Can you work these out from the model? Positions are in its coordinate system, mm. A direction names the side the tool comes from. Round coordinates to 2 decimals unless told otherwise and drop trailing zeros. One line per question, with ' | ' between items.
```python
from build123d import *

# Parameters (mm, degrees)
SKETCH1_R           = 2.5
BOSS_EXTRUDE1_DEPTH = 200


with BuildPart() as part:
    # Sketch1 → Boss-Extrude1 (new body)
    with BuildSketch(Plane(origin=(0, 0, -25), x_dir=(-1, 0, 0), z_dir=(0, 0, -1))):
        with BuildLine():
            Line((12.5, 4.32), (12.5, 10.537068835))
            ThreePointArc((12.5, 10.537068835), (11.925070773, 11.925070773), (10.537068835, 12.5))
            Line((10.537068835, 12.5), (4.32, 12.5))
            ThreePointArc((4.32, 12.5), (3.25, 11.43), (4.32, 10.36))
            Line((4.32, 10.36), (6.42, 10.36))
            ThreePointArc((6.42, 10.36), (7.35325999, 9.736168088), (7.133653911, 8.635298598))
            Line((7.133653911, 8.635298598), (3.795290766, 5.301828272))
            ThreePointArc((3.795290766, 5.301828272), (2.76743922, 4.61585726), (1.555406707, 4.375))
            Line((1.555406707, 4.375), (-1.555406707, 4.375))
            ThreePointArc((-1.555406707, 4.375), (-2.76743922, 4.61585726), (-3.795290766, 5.301828272))
            Line((-3.795290766, 5.301828272), (-7.133653912, 8.635298598))
            ThreePointArc((-7.133653912, 8.635298598), (-7.35325999, 9.736168088), (-6.42, 10.36))
            Line((-6.42, 10.36), (-4.32, 10.36))
            ThreePointArc((-4.32, 10.36), (-3.25, 11.43), (-4.32, 12.5))
            Line((-4.32, 12.5), (-10.537068835, 12.5))
            ThreePointArc((-10.537068835, 12.5), (-11.925070773, 11.925070773), (-12.5, 10.537068835))
            Line((-12.5, 10.537068835), (-12.5, 4.32))
            ThreePointArc((-12.5, 4.32), (-11.43, 3.25), (-10.36, 4.32))
            Line((-10.36, 4.32), (-10.36, 6.396886949))
            ThreePointArc((-10.36, 6.396886949), (-9.736852394, 7.329863489), (-8.636346088, 7.111588351))
            Line((-8.636346088, 7.111588351), (-5.432204773, 3.912143135))
            ThreePointArc((-5.432204773, 3.912143135), (-4.708985779, 2.831057106), (-4.455, 1.555406707))
            Line((-4.455, 1.555406707), (-4.455, -1.555406707))
            ThreePointArc((-4.455, -1.555406707), (-4.708985779, -2.831057106), (-5.432204773, -3.912143135))
            Line((-5.432204773, -3.912143135), (-8.636346088, -7.111588351))
            ThreePointArc((-8.636346088, -7.111588351), (-9.736852394, -7.329863489), (-10.36, -6.396886949))
            Line((-10.36, -6.396886949), (-10.36, -4.32))
            ThreePointArc((-10.36, -4.32), (-11.43, -3.25), (-12.5, -4.32))
            Line((-12.5, -4.32), (-12.5, -10.537068835))
            ThreePointArc((-12.5, -10.537068835), (-11.925070773, -11.925070773), (-10.537068835, -12.5))
            Line((-10.537068835, -12.5), (-4.387856959, -12.5))
            ThreePointArc((-4.387856959, -12.5), (-3.317856959, -11.43), (-4.387856959, -10.36))
            Line((-4.387856959, -10.36), (-6.42, -10.36))
            ThreePointArc((-6.42, -10.36), (-7.35325999, -9.736168088), (-7.133653912, -8.635298598))
            Line((-7.133653912, -8.635298598), (-3.795290766, -5.301828272))
            ThreePointArc((-3.795290766, -5.301828272), (-2.76743922, -4.61585726), (-1.555406707, -4.375))
            Line((-1.555406707, -4.375), (1.555406707, -4.375))
            ThreePointArc((1.555406707, -4.375), (2.76743922, -4.61585726), (3.795290766, -5.301828272))
            Line((3.795290766, -5.301828272), (7.133653912, -8.635298598))
            ThreePointArc((7.133653912, -8.635298598), (7.35325999, -9.736168088), (6.42, -10.36))
            Line((6.42, -10.36), (4.387856959, -10.36))
            ThreePointArc((4.387856959, -10.36), (3.317856959, -11.43), (4.387856959, -12.5))
            Line((4.387856959, -12.5), (10.537068835, -12.5))
            ThreePointArc((10.537068835, -12.5), (11.925070773, -11.925070773), (12.5, -10.537068835))
            Line((12.5, -10.537068835), (12.5, -4.32))
            ThreePointArc((12.5, -4.32), (11.43, -3.25), (10.36, -4.32))
            Line((10.36, -4.32), (10.36, -6.396886949))
            ThreePointArc((10.36, -6.396886949), (9.736852394, -7.329863489), (8.636346088, -7.111588351))
            Line((8.636346088, -7.111588351), (5.432204773, -3.912143135))
            ThreePointArc((5.432204773, -3.912143135), (4.708985779, -2.831057106), (4.455, -1.555406707))
            Line((4.455, -1.555406707), (4.455, 1.555406707))
            ThreePointArc((4.455, 1.555406707), (4.708985779, 2.831057106), (5.432204773, 3.912143135))
            Line((5.432204773, 3.912143135), (8.636346088, 7.111588351))
            ThreePointArc((8.636346088, 7.111588351), (9.736852394, 7.329863489), (10.36, 6.396886949))
            Line((10.36, 6.396886949), (10.36, 4.32))
            ThreePointArc((10.36, 4.32), (11.43, 3.25), (12.5, 4.32))
        make_face()
        with Locations(Location((0, 0, 0), (0, 0, 180))):
            Circle(SKETCH1_R, mode=Mode.SUBTRACT)
    extrude(amount=-BOSS_EXTRUDE1_DEPTH)


solid = part.part
```
(1) Will these pins go through, and if not, where does the flat tip stop? pin 1 Ø1.6 at (x, z) = (0, 75.5) entering from -Y (3 decimals); pin 2 Ø0.9 at (y, z) = (0.5, 97) entering from +X (3 decimals); pin 3 Ø1.6 at (y, z) = (0.5, 47) entering from -X (3 decimals).
Final values:
pin 1: y = -4.375 | pin 2: x = 4.455 | pin 3: x = -4.455
(2) Please list where these lines run through material, in increasing order: probe 1 along Y at (x, z) = (0, 69) (3 decimals); probe 2 along X at (y, z) = (6.5, 95); probe 3 along X at (y, z) = (6, 152). Write a range as [from, to].
Final values:
probe 1: [-4.375, -2.5], [2.5, 4.375] | probe 2: [-12.5, -10.35], [-8.02, -5], [5, 8.02], [10.35, 12.5] | probe 3: [-12.5, -10.36], [-7.52, -4.49], [4.49, 7.52], [10.36, 12.5]
(3) On a 3-axis mill with a long thin cutter (end or side, diameter ignored), from which of +Z, -Z, +X, -X, +Y, -Y can I reach the whole of each face in a straight line? I mean faces 4 (the flat face through (7.01, -5.49, 73.6)), 5 (the flat face through (0, 4.375, 74)), 6 (the flat face through (-7, -12.5, 74)), 7 (the flat face through (0, -4.375, 74)). Say none if no direction works.
Final values:
face 4: +Z, -Z | face 5: +Z, -Z, +Y | face 6: +Z, -Z, +X, -X, -Y | face 7: +Z, -Z, -Y
(4) Thinking about a two-plate mould opening in Y: for faces 1 (the flat face through (12.5, -7, 74)), 2 (the flat face through (8, -12.5, 74)), 3 (the flat face through (5.488, -6.992, 73.6)), which applies, released by +Y, released by -Y, zero draft, split by the parting line, or undercut?
Final values:
face 1: zero draft | face 2: released by -Y | face 3: undercut
